Source: CAD feature listing. Evaluate the final solid. Frame: model axes, mm. A direction names the side the tool comes from. Round coordinates to 2 decimals unless told otherwise and drop trailing zeros. Write each loop counter-clockwise with the first axis right and the second up, starting at its lowest first coordinate (ties: lowest second). Pieces come first, ordered by that corner, then holes. Notation, with made-up numbers: M 83,-20 L 138,-20 A21 ccw 138,1 Z; hole C -39.5,-19.5 d11. An arc over 180 degrees is marked long. Answer in a Markdown table with one row per item. Add a question column.
Item 1: Material intervals for probe 1 along X at (y, z) = (-8.5, 33); probe 2 along Z at (x, y) = (29, -12.5); probe 3 along Z at (x, y) = (6.5, 1), sorted ascending.
Item 2: Cut plane A-A on z = 3.5. Return loops of the section in (x, y) (3 decimals), and give its area (3 significant figures).
Item 3: Contact query for flat-ended pins moving along their axis: pin 1 (1 mm diameter, centred on x = -20.5, z = 12.5, fed in from -Y); pin 2 (10 mm diameter, centred on y = 5.5, z = 29.5, fed in from +X); pin 3 (8 mm diameter, centred on x = 12.5, z = 16.5, fed in from +Y). Output: stop coordinate, or through.
Item 4: Cut plane C-C on x = -31.5. Return loops of the section in (y, z).
Item 5: Set-up query: faces 1 (the face through (36.145, 2.861, 6.261)), 2 (the face through (-52.23, 2.21, 30.69)), 3 (the face through (5, 0, 25.4)). Return all of +Z, -Z, +X, -X, +Y, -Y with unobstructed straight access to the full face (end or side cutting, diameter ignored); none if empty.
Item 6: Cut plane B-B on y = 8. Return loops of the section in (x, z), and give its area (3 significant figures).
Item 7: Cut plane D-D on z = 14.5. Return loops of the section in (x, y) (3 decimals).
from build123d import *

# Parameters (mm, degrees)
F0_R     = 15.875
F1_DEPTH = 50.8
F2_DEPTH = 25.4
F0_R_2   = 9.525
F3_DEPTH = 12.7
F4_R     = 6.35


with BuildPart() as f1:
    # F0 (on Top) → F1 (new body)
    with BuildSketch(Plane.XY):
        with BuildLine():
            ThreePointArc((4.8347544076, 0), (-1.5460097383, 17.998514379), (-17.8386678043, 27.9589342538))
            ThreePointArc((-17.8386678043, 27.9589342538), (-52.3151461351, 0.07539214), (-17.9862828844, -27.9896862818))
            ThreePointArc((-17.9862828844, -27.9896862818), (-1.5935741791, -18.0570088971), (4.8347544076, 0))
        make_face()
        with Locations((-23.7402455924, 0)):
            Circle(F0_R, mode=Mode.SUBTRACT)
    extrude(amount=F1_DEPTH)

    # F0 (on Top) → F2 (join)
    with BuildSketch(Plane.XY):
        with BuildLine():
            ThreePointArc((25.7271171156, -19.0033307041), (8.0139347128, -0.3990640994), (24.9322885076, 18.9308316998))
            Line((24.9322885076, 18.9308316998), (-17.8386678043, 27.9589342538))
            ThreePointArc((-17.8386678043, 27.9589342538), (-1.5460097383, 17.998514379), (4.8347544076, 0))
            ThreePointArc((4.8347544076, 0), (-1.5935741791, -18.0570088971), (-17.9862828844, -27.9896862818))
            Line((-17.9862828844, -27.9896862818), (25.7271171156, -19.0033307041))
        make_face()
    extrude(amount=F2_DEPTH)

    # F0 (on Top) → F3 (join)
    with BuildSketch(Plane.XY):
        with BuildLine():
            ThreePointArc((25.7271171156, -19.0033307041), (40.0504387542, -13.9335788729), (46.1097544076, 0))
            ThreePointArc((46.1097544076, 0), (39.7557040492, 14.2026533682), (24.9322885076, 18.9308316998))
            ThreePointArc((24.9322885076, 18.9308316998), (8.0139347128, -0.3990640994), (25.7271171156, -19.0033307041))
        make_face()
        with Locations((27.0597544076, 0)):
            Circle(F0_R_2, mode=Mode.SUBTRACT)
    extrude(amount=F3_DEPTH)

    # F4
    f4_edges = [f1.edges().sort_by_distance(p)[0] for p in [
        (25.727117, -19.003331, 19.05),
        (24.932289, 18.930832, 19.05),
    ]]
    fillet(f4_edges, radius=F4_R)


solid = f1.part
Results below:
| question | item | result |
|---|---|---|
| 1 | probe 1 | -51.02 to -37.15, -10.33 to 3.54 |
| 1 | probe 2 | 0 to 12.7 |
| 1 | probe 3 | 0 to 25.4 |
| 2 | outline | M -17.986,-27.99 L 25.727,-19.003 A19.05 ccw long 24.932,18.931 L -17.839,27.959 A28.575 ccw long Z; hole C -23.74,0 d31.75; hole C 27.06,0 d19.05 |
| 2 | area | 3,200 mm2 |
| 3 | pin 1 | y = -28.44 |
| 3 | pin 2 | x = 9.94 |
| 3 | pin 3 | y = 22.4 |
| 4 | outline | M -27.5,0 L -13.85,0 L -13.85,50.8 L -27.5,50.8 Z; M 13.85,0 L 27.5,0 L 27.5,50.8 L 13.85,50.8 Z |
| 5 | face 1 | +Z, -Z |
| 5 | face 2 | +Z |
| 5 | face 3 | +Z, +X |
| 6 | outline | M -51.17,0 L -37.45,0 L -37.45,50.8 L -51.17,50.8 Z; M -10.03,0 L 21.89,0 L 21.89,12.7 L 9.77,12.7 L 9.77,25.4 L 3.69,25.4 L 3.69,50.8 L -10.03,50.8 Z; M 32.23,0 L 44.35,0 L 44.35,12.7 L 32.23,12.7 Z |
| 6 | area | 1,860 mm2 |
| 7 | outline | M -17.986,-27.99 L 8.824,-22.478 A6.35 ccw 12.424,-12.194 A19.05 cw 12.346,12.1 A6.35 ccw 8.753,22.346 L -17.839,27.959 A28.575 ccw long Z; hole C -23.74,0 d31.75 |
